```python
from build123d import *

# Parameters (mm, degrees)
F0_R     = 3.3
F1_DEPTH = 4
F2_D     = 6.6


with BuildPart() as f1:
    # F0 (on Top) → F1 (new body)
    with BuildSketch(Plane.XY):
        with BuildLine():
            ThreePointArc((34.0567992704, 89.8965680339), (40.7519566994, 94.3854046152), (36.9381754792, 101.4868030449))
            ThreePointArc((36.9381754792, 101.4868030449), (0, 108), (-36.9381754792, 101.4868030449))
            ThreePointArc((-36.9381754792, 101.4868030449), (-40.7070213733, 94.393880651), (-34.0444122932, 89.9079707427))
            ThreePointArc((-34.0444122932, 89.9079707427), (-32.0231312915, 89.4750579815), (-30.7617113386, 87.8374346888))
            Line((-30.7617113386, 87.8374346888), (-29.240736677, 82.9998754131))
            ThreePointArc((-29.240736677, 82.9998754131), (-25.1204073514, 90.5812626016), (-17.6838927225, 86.2048718935))
            Line((-17.6838927225, 86.2048718935), (-18.8216514871, 90.9271435562))
            ThreePointArc((-18.8216514871, 90.9271435562), (-18.4124399871, 93.2770471476), (-16.4181773429, 94.585640838))
            ThreePointArc((-16.4181773429, 94.585640838), (-12.9456893063, 95.1231261491), (-9.455857384, 95.533170999))
            ThreePointArc((-9.455857384, 95.533170999), (-7.1844187157, 94.8051137786), (-6.1621056327, 92.6500321326))
            Line((-6.1621056327, 92.6500321326), (-5.9965124161, 87.7954545455))
            ThreePointArc((-5.9965124161, 87.7954545455), (-0.1022875924, 93.9991280407), (6, 88))
            ThreePointArc((6, 88), (5.9991280407, 87.8977124076), (5.9965124161, 87.7954545455))
            Line((5.9965124161, 87.7954545455), (6.1621056327, 92.6500321326))
            ThreePointArc((6.1621056327, 92.6500321326), (7.1844187157, 94.8051137786), (9.455857384, 95.533170999))
            ThreePointArc((9.455857384, 95.533170999), (12.9456893063, 95.1231261491), (16.4181773429, 94.585640838))
            ThreePointArc((16.4181773429, 94.585640838), (18.4124399871, 93.2770471476), (18.8216514871, 90.9271435562))
            Line((18.8216514871, 90.9271435562), (17.6838927225, 86.2048718935))
            ThreePointArc((17.6838927225, 86.2048718935), (24.224611805, 90.7576048489), (29.5169770949, 84.7994798824))
            ThreePointArc((29.5169770949, 84.7994798824), (29.4475149075, 83.8891385982), (29.240736677, 82.9998754131))
            Line((29.240736677, 82.9998754131), (30.7588194113, 87.8282367253))
            ThreePointArc((30.7588194113, 87.8282367253), (32.026773101, 89.4699693779), (34.0567992704, 89.8965680339))
        make_face()
        with BuildLine():
            ThreePointArc((-35.9121150493, 98.6677251825), (-1e-10, 105), (35.9121150492, 98.6677251825))
            ThreePointArc((35.9121150492, 98.6677251825), (37.7051324816, 94.8225868902), (33.8599941892, 93.0295694578))
            ThreePointArc((33.8599941892, 93.0295694578), (-1e-10, 99), (-33.8599941894, 93.0295694578))
            ThreePointArc((-33.8599941892, 93.0295694574), (-37.7051324816, 94.8225868898), (-35.9121150492, 98.6677251821))
        make_face(mode=Mode.SUBTRACT)
        with BuildLine():
            ThreePointArc((-5.9965124161, 87.7954545455), (0, 82), (5.9965124161, 87.7954545455))
            ThreePointArc((5.9965124161, 87.7954545455), (5.9991280407, 87.8977124076), (6, 88))
            ThreePointArc((6, 88), (-0.1022875924, 93.9991280407), (-5.9965124161, 87.7954545455))
        make_face()
        with Locations((0, 88)):
            Circle(F0_R, mode=Mode.SUBTRACT)
        with BuildLine():
            ThreePointArc((17.6838927225, 86.2048718935), (21.9135468384, 79.0176971631), (29.240736677, 82.9998754131))
            ThreePointArc((29.240736677, 82.9998754131), (29.4475149075, 83.8891385982), (29.5169770949, 84.7994798824))
            ThreePointArc((29.5169770949, 84.7994798824), (24.224611805, 90.7576048489), (17.6838927225, 86.2048718935))
        make_face()
        with Locations((23.5169770949, 84.7994798824)):
            Circle(F0_R, mode=Mode.SUBTRACT)
        with BuildLine():
            ThreePointArc((-17.6838927225, 86.2048718935), (-25.1204073514, 90.5812626016), (-29.240736677, 82.9998754131))
            ThreePointArc((-29.240736677, 82.9998754131), (-22.6066358108, 78.8689420698), (-17.5169770949, 84.7994798824))
            ThreePointArc((-17.5169770949, 84.7994798824), (-17.5588521283, 85.5071145925), (-17.6838927225, 86.2048718935))
        make_face()
        with Locations((-23.5169770949, 84.7994798824)):
            Circle(F0_R, mode=Mode.SUBTRACT)
        with Locations((0, 88)):
            Circle(F0_R)
        with Locations((23.5169770949, 84.7994798824)):
            Circle(F0_R)
        with Locations((-23.5169770949, 84.7994798824)):
            Circle(F0_R)
    extrude(amount=F1_DEPTH)

    # F2 (through all)
    with Locations(Plane(origin=(0, 0, 0), x_dir=(1, 0, 0), z_dir=(0, 0, -1))):
        with Locations((-23.5169770949, -84.7994798824), (0, -88), (23.5169770949, -84.7994798824)):
            Hole(F2_D / 2)


solid = f1.part
```
Check sheet for the modelled part. Datum: model origin and axes. Units: mm. A direction names the side the tool comes from. Give positions to 0.01 mm unless a question says otherwise; leave off trailing zeros. Order: outer loops, then holes, each group sorted by start corner. A loop starts at its lowest first (then second) coordinate and runs counter-clockwise, first axis right, second up. Notation, with made-up numbers: (73.25, 63) -> (103.25, 63) arc R22 cw to (103.25, 78) -> close; hole circle Ø11 at (29, 65). An arc over 180 degrees is marked (long way). Use CSV: the item, a comma, the result in double quotes. Start each with the question number.
1) Mould release check, pull along Y, two halves, no side actions. Record for faces 4 (the face through (-1, 94, 4)), 5 (the face through (0, 99, 2)), 6 (the face through (-32.05, 89.49, 1.97)): released by +Y, released by -Y, zero draft, split by the parting line, or undercut.
2) Go/stop test with flat-tipped pins: P1, Ø1.5, axis at x = -31.5, y = 96, coming from the +Z side; P2, Ø2, axis at x = -31, z = 1, coming from the +Y side; P3, Ø2, axis at x = 26.5, z = 3, coming from the +Y side. Record where each tip stops, or that it passes through.
3) Sectioned sample at D-D, the plane y = 83.75. Record the boundary of the cut face in (x, z).
4) Material ranges on line 1 (Y direction, x = -23, z = 1.45); line 2 (X direction, y = 90.5, z = 1.25); line 3 (X direction, y = 82.75, z = 2.9), recorded low to high. Write a range as from..to.
5) Sectioned sample at C-C, the plane x = -15. Record the boundary of the cut face in (y, z), plus the area to 3 significant figures.
6) Sectioned sample at B-B, the plane y = 104. Record the boundary of the cut face in (x, z).
7) Set-up check for faces 1 (the face through (-12.994, 95.116, 1.972)), 2 (the face through (29.99, 85.38, 1.97)), 3 (the face through (-0.5, 105, 2)): record each of +Z, -Z, +X, -X, +Y, -Y from which the full face is reachable in a straight line by a thin tool's end or side.
8) Sectioned sample at A-A, the plane x = 0. Record the boundary of the cut face in (y, z).
Recorded:
1,face 4,"zero draft"
1,face 5,"undercut"
1,face 6,"released by -Y"
2,P1,"through"
2,P2,"y = 103.75"
2,P3,"y = 104.95"
3,outline,"(-29.48, 0) -> (-26.65, 0) -> (-26.65, 4) -> (-29.48, 4) -> close; (-20.39, 0) -> (-17.61, 0) -> (-17.61, 4) -> (-20.39, 4) -> close; (-4.24, 0) -> (4.24, 0) -> (4.24, 4) -> (-4.24, 4) -> close; (17.61, 0) -> (20.39, 0) -> (20.39, 4) -> (17.61, 4) -> close; (26.65, 0) -> (29.48, 0) -> (29.48, 4) -> (26.65, 4) -> close"
4,line 1,"78.82..81.54, 88.06..96.29, 102.45..105.52"
4,line 2,"-37.6..-18.72, -6.09..-2.15, 2.15..6.09, 18.72..37.68"
4,line 3,"-29.16..-26.1, -20.93..-17.88, -2.9..2.9, 17.88..20.93, 26.1..29.16"
5,outline,"(94.82, 0) -> (97.86, 0) -> (97.86, 4) -> (94.82, 4) -> close; (103.92, 0) -> (106.95, 0) -> (106.95, 4) -> (103.92, 4) -> close"
5,area,"24.3 mm2"
6,outline,"(-29.12, 0) -> (-14.46, 0) -> (-14.46, 4) -> (-29.12, 4) -> close; (14.46, 0) -> (29.12, 0) -> (29.12, 4) -> (14.46, 4) -> close"
7,face 1,"+Z, -Z, -Y"
7,face 2,"+Z, -Z, +X, -Y"
7,face 3,"+Z, -Z"
8,outline,"(82, 0) -> (84.7, 0) -> (84.7, 4) -> (82, 4) -> close; (91.3, 0) -> (99, 0) -> (99, 4) -> (91.3, 4) -> close; (105, 0) -> (108, 0) -> (108, 4) -> (105, 4) -> close"
